Autodesk Inventor part; units mm, degrees
ref_plane "YZ Plane" through (0, 0, 0) normal (1, 0, 0) x (0, 1, 0)
ref_plane "XZ Plane" through (0, 0, 0) normal (0, 1, 0) x (-1, 0, 0)
ref_plane "XY Plane" through (0, 0, 0) normal (0, 0, 1) x (1, 0, 0)
sketch "Sketch1" plane through (0, 0, 0) normal (0, 0, 1) x (1, 0, 0)
  line L0 (0, 57.1566) -> (0, -74.2716) construction
  line L1 (-84, 0) -> (84, 0) construction
  line L2 (-60, 30) -> (60, 30)
  line L3 (60, 30) -> (60, -30)
  line L4 (60, -30) -> (-60, -30)
  line L5 (-60, -30) -> (-60, 30)
  point P0 (0, 0)
  dimension "d0" = 120
  dimension "d1" = 60
extrude "Extrusion1" add sketch "Sketch1" along normal blind 24
sketch "Sketch2" plane through (-60, -30, 0) normal (0, -1, 0) x (1, 0, 0)
  line L0 (120, 24) -> (0, 24)
  line L1 (60, 28.8) -> (60, -4.8) construction
  line L2 (-24, 0) -> (144, 0) construction
  line L3 (41.9586, 17) -> (78.0414, 17) construction
  line L4 (41.9586, 17) -> (46.0001, 24) construction
  line L5 (41.9586, 17) -> (50.0416, 17) construction
  line L6 (78.0414, 17) -> (63.0829, 17) construction
  line L7 (73.9999, 24) -> (46.0001, 24) construction
  line L8 (73.9999, 24) -> (78.0414, 17)
  line L9 (78.0414, 17) -> (40, 17)
  line L10 (40, 17) -> (40, 24)
  line L11 (73.9999, 24) -> (40, 24)
  point P0 (60, 0)
  point P1 (77.464, 18)
  dimension "d5" = 60
  dimension "d7" = 7
  dimension "d37" = 1
  dimension "d39" = 17.464
  dimension "d40" = 60
  dimension "d64" = 20
extrude "Extrusion2" cut sketch "Sketch2" against normal up to next
sketch "Sketch9" plane through (0, 0, 24) normal (0, 0, 1) x (1, 0, 0)
  line L0 (0, 57.1566) -> (0, -74.2716) construction
  line L1 (-84, 0) -> (84, 0) construction
  line L2 (25, 37.3826) -> (25, -38.2478) construction
  line L3 (50, 36.5596) -> (50, -55.4961) construction
  line L4 (-25, 38.3811) -> (-25, -39.94) construction
  line L5 (-50, 35.8185) -> (-50, -44.962) construction
  line L6 (-20, -30) -> (-20, 30) construction
  line L7 (-60, 30) -> (-20, 30) construction
  line L8 (-60, -30) -> (-60, 30) construction
  line L9 (-20, -30) -> (-60, -30) construction
  line L10 (13.9999, 30) -> (13.9999, -30) construction
  line L11 (60, -30) -> (13.9999, -30) construction
  line L12 (60, 30) -> (60, -30) construction
  line L13 (13.9999, 30) -> (60, 30) construction
  line L14 (60, -30) -> (-60, -30)
  line L15 (-60, 30) -> (-35, 30)
  line L16 (-35, 30) -> (-35, -30)
  line L17 (-35, -30) -> (-60, -30)
  line L18 (-60, -30) -> (-60, 30)
  line L19 (13.9999, 30) -> (60, 30)
  line L20 (60, -30) -> (13.9999, -30)
  line L21 (60, 30) -> (35, 30)
  line L22 (35, 30) -> (35, -30)
  line L23 (35, -30) -> (60, -30)
  line L24 (60, -30) -> (60, 30)
  point P0 (0, 0)
  dimension "d65" = 25
  dimension "d66" = 25
  dimension "d67" = 25
  dimension "d68" = 25
  dimension "d69" = 25
  dimension "d70" = 25
extrude "Extrusion7" cut sketch "Sketch9" against normal blind 14
sketch "Sketch10" plane through (0, 0, 10) normal (0, 0, 1) x (1, 0, 0)
  line L0 (-60, -30) -> (-60, 30) construction
  line L1 (-35, -30) -> (-60, -30) construction
  line L2 (-35, 30) -> (-35, -30) construction
  line L3 (-60, 30) -> (-35, 30) construction
  line L4 (60, -30) -> (35, -30) construction
  line L5 (60, 30) -> (60, -30) construction
  line L6 (35, 30) -> (60, 30) construction
  line L7 (35, -30) -> (35, 30) construction
  line L8 (-88.2, 0) -> (88.2, 0) construction
  line L9 (0, 42) -> (0, -42) construction
  line L10 (-60, -30) -> (-60, 30) construction
  line L11 (-60, 12.5) -> (60, 12.5) construction
  line L12 (60, 30) -> (60, -30) construction
  line L13 (-60, -12.5) -> (60, -12.5) construction
  line L14 (-60, 12.5) -> (-40, 12.5) construction
  line L15 (-60, 9.5) -> (-40, 9.5)
  line L16 (-40, 15.5) -> (-60, 15.5)
  arc A0 (-60, 15.5) -> (-60, 9.5) centre (-60, 12.5) ccw
  arc A1 (-40, 9.5) -> (-40, 15.5) centre (-40, 12.5) ccw
  line L17 (-60, -12.5) -> (-40, -12.5) construction
  line L18 (-60, -15.5) -> (-40, -15.5)
  line L19 (-40, -9.5) -> (-60, -9.5)
  arc A2 (-60, -9.5) -> (-60, -15.5) centre (-60, -12.5) ccw
  arc A3 (-40, -15.5) -> (-40, -9.5) centre (-40, -12.5) ccw
  line L20 (60, 12.5) -> (40, 12.5) construction
  line L21 (60, 15.5) -> (40, 15.5)
  line L22 (40, 9.5) -> (60, 9.5)
  arc A4 (60, 9.5) -> (60, 15.5) centre (60, 12.5) ccw
  arc A5 (40, 15.5) -> (40, 9.5) centre (40, 12.5) ccw
  line L23 (60, -12.5) -> (40, -12.5) construction
  line L24 (60, -9.5) -> (40, -9.5)
  line L25 (40, -15.5) -> (60, -15.5)
  arc A6 (60, -15.5) -> (60, -9.5) centre (60, -12.5) ccw
  arc A7 (40, -9.5) -> (40, -15.5) centre (40, -12.5) ccw
  point P0 (0, 0)
  point P1 (-50, 12.5)
  point P2 (-50, -12.5)
  point P3 (50, 12.5)
  point P4 (50, -12.5)
  dimension "d73" = 12.5
  dimension "d74" = 12.5
  dimension "d75" = 6
  dimension "d76" = 20
  dimension "d77" = 6
  dimension "d78" = 20
  dimension "d79" = 6
  dimension "d80" = 20
  dimension "d81" = 6
  dimension "d82" = 20
extrude "Extrusion8" cut sketch "Sketch10" against normal up to next
sketch "Sketch11" plane through (-35, -30, 24) normal (-1, 0, 0) x (0, 0, 1)
  line L0 (-7, 0) -> (-7, 60) construction
  line L1 (0, 60) -> (0, 0) construction
  line L2 (-14, 60) -> (0, 60) construction
  line L3 (-14, 60) -> (-14, 0) construction
  line L4 (0, 0) -> (-14, 0) construction
  line L5 (-3.5, 60) -> (-3.5, 0) construction
  line L6 (0, 0) -> (-14, 0) construction
  point P0 (-24, 30)
  point P1 (-3.5, 7.5)
  point P2 (-3.5, 22.5)
  point P3 (-3.5, 37.5)
  point P4 (-3.5, 52.5)
  dimension "d85" = 3.5
  dimension "d86" = 7.5
  dimension "d87" = 15
  dimension "d88" = 15
  dimension "d89" = 15
hole "Hole3" at (-35, -22.5, 20.5) at (-35, -7.5, 20.5) at (-35, 7.5, 20.5) at (-35, 22.5, 20.5) direction (1, 0, 0) diameter 3.242 end up to surface
properties part number "MVX-10-Bracket-V5"
Geometry check sheet. Reference: the model listing, model coordinates, mm. A direction names the side the tool comes from. Give positions to 0.01 mm unless a question says otherwise; leave off trailing zeros. Loops run counter-clockwise (first coordinate to the right, second up) from the corner with the lowest first, then second, coordinate; pieces in that order, holes last. Notation, with made-up numbers: (-21.75, -31.5) - (-0.75, -31.5) arc R23 cw to (-0.75, -9.5) - close; hole circle Ø4 at (5.5, 59). An arc over 180 degrees is marked (long way). Use CSV: the item, a comma, the result in double quotes. Start each with the question number.
Q1. Go/stop test with flat-tipped pins: pin 1 Ø3.5 at (y, z) = (22.5, 20.5) entering from +X; pin 2 Ø1.5 at (x, y) = (-36.5, -16) entering from +Z; pin 3 Ø12 at (x, y) = (-5.5, -4.5) entering from +Z. Record where each tip stops, or that it passes through.
Q2. Scan lines: probe 1 along Y at (x, z) = (-23.75, 20.5); probe 2 along Z at (x, y) = (-31.5, 7.5); probe 3 along X at (y, z) = (24, 12.5). Record each from-to range of solid material in increasing order. Write a range as from..to.
Q3. Access from +Z, -Z, +X, -X, +Y, -Y to the whole of each face (thin tool, end or side, straight path). Record for faces 5 (the face through (-27.395, -7.987, 22.046)), 6 (the face through (15.99, -0.42, 20.55)), 7 (the face through (47, 0, 10)).
Q4. Section check A-A, the plane x = -44. Record the cut outline in (y, z).
Q5. Section check D-D, the plane z = 8.25. Record the cut outline in (x, y), and give its area (3 significant figures).
Q6. Section check B-B, the plane y = -22.5. Record the cut outline in (x, z), and give its area (3 significant figures).
Q7. Release check for a two-part mould opening along X. For faces 1 (the face through (-37, -12.6, 5.1)), 2 (the face through (35, 0, 17)), 3 (the face through (-20, 0, 20)), 4 (the face through (-50, -9.5, 5)) record: +X half, -X half, draft (parallel to the pull), parting line (faces both ways), or undercut.
Q8. Section check C-C, the plane x = -26. Record the cut outline in (y, z).
Findings below:
1,pin 1,"stops at x = 35"
1,pin 2,"stops at z = 10"
1,pin 3,"stops at z = 17"
2,probe 1,"y = -30..-24.12, -20.88..-9.12, -5.88..5.88, 9.12..20.88, 24.12..30"
2,probe 2,"z = 0..18.88, 22.12..24"
2,probe 3,"x = -35..35"
3,face 5,"-X"
3,face 6,"+Y, -Y"
3,face 7,"+Z, +X, +Y, -Y"
4,outline,"(-30, 0) - (-15.5, 0) - (-15.5, 10) - (-30, 10) - close; (-9.5, 0) - (9.5, 0) - (9.5, 10) - (-9.5, 10) - close; (15.5, 0) - (30, 0) - (30, 10) - (15.5, 10) - close"
5,outline,"(-60, -30) - (60, -30) - (60, -15.5) - (40, -15.5) arc R3 cw to (40, -9.5) - (60, -9.5) - (60, 9.5) - (40, 9.5) arc R3 cw to (40, 15.5) - (60, 15.5) - (60, 30) - (-60, 30) - (-60, 15.5) - (-40, 15.5) arc R3 cw to (-40, 9.5) - (-60, 9.5) - (-60, -9.5) - (-40, -9.5) arc R3 cw to (-40, -15.5) - (-60, -15.5) - close"
5,area,"6,660 mm^2"
6,outline,"(-60, 0) - (60, 0) - (60, 10) - (35, 10) - (35, 24) - (14, 24) - (18.04, 17) - (-20, 17) - (-20, 18.88) - (-35, 18.88) - (-35, 10) - (-60, 10) - close; (-35, 22.12) - (-20, 22.12) - (-20, 24) - (-35, 24) - close"
6,area,"1,880 mm^2"
7,face 1,"-X half"
7,face 2,"+X half"
7,face 3,"undercut"
7,face 4,"draft"
8,outline,"(-30, 0) - (30, 0) - (30, 24) - (-30, 24) - close; hole circle Ø3.24 at (-22.5, 20.5); hole circle Ø3.24 at (-7.5, 20.5); hole circle Ø3.24 at (7.5, 20.5); hole circle Ø3.24 at (22.5, 20.5)"
